Source: CAD feature listing. Evaluate the final solid. Frame: model axes, mm. A direction names the side the tool comes from. Round coordinates to 2 decimals unless told otherwise and drop trailing zeros. Write each loop counter-clockwise with the first axis right and the second up, starting at its lowest first coordinate (ties: lowest second). Pieces come first, ordered by that corner, then holes.
```python
from build123d import *

# Parameters (mm, degrees)
AUFSATZ_LINEAR_AUSTRAGEN1_DEPTH      = 10
AUFSATZ_LINEAR_AUSTRAGEN2_DEPTH      = 30
SCHNITT_LINEAR_AUSTRAGEN1_DEPTH      = 80.274901172
SCHNITT_LINEAR_AUSTRAGEN1_DEPTH_BACK = 80.274901172
SCHNITT_LINEAR_AUSTRAGEN2_DEPTH      = 47.124758374
SCHNITT_LINEAR_AUSTRAGEN2_DEPTH_BACK = 47.124758374
DURCHGANGSLOCH_F_R_M81_D             = 9
M12_GEWINDEBOHRUNG1_D                = 10.2


with BuildPart() as part:
    # Skizze1 → Aufsatz-Linear austragen1 (new body)
    with BuildSketch(Plane(origin=(0, 0, 0), x_dir=(1, 0, 0), z_dir=(0, 1, 0))):
        with BuildLine():
            Line((-69.274901172, 46.124758374), (69.274901172, 46.124758374))
            ThreePointArc((69.274901172, 46.124758374), (76.345968983, 43.195826186), (79.274901172, 36.124758374))
            Line((79.274901172, 36.124758374), (79.274901172, -36.124758374))
            ThreePointArc((79.274901172, -36.124758374), (76.345968983, -43.195826186), (69.274901172, -46.124758374))
            Line((69.274901172, -46.124758374), (-69.274901172, -46.124758374))
            ThreePointArc((-69.274901172, -46.124758374), (-76.345968983, -43.195826186), (-79.274901172, -36.124758374))
            Line((-79.274901172, -36.124758374), (-79.274901172, 36.124758374))
            ThreePointArc((-79.274901172, 36.124758374), (-76.345968983, 43.195826186), (-69.274901172, 46.124758374))
        make_face()
    extrude(amount=AUFSATZ_LINEAR_AUSTRAGEN1_DEPTH)

    # Skizze2 → Aufsatz-Linear austragen2 (add, symmetric)
    with BuildSketch(Plane.XY):
        Polygon((-30.968636567, 51.19380308), (-44.314952745, 10), (44.314952745, 10), (30.968636567, 51.19380308), align=None)
    extrude(amount=AUFSATZ_LINEAR_AUSTRAGEN2_DEPTH, both=True)

    # Skizze3 → Schnitt-Linear austragen1 (cut, two sides)
    with BuildSketch(Plane(origin=(0, 0, 0), x_dir=(0, 0, -1), z_dir=(1, 0, 0))) as schnitt_linear_austragen1_sk:
        Polygon((-30, 10), (-22.945404255, 51.19380308), (-30, 51.19380308), align=None)
        Polygon((30, 51.19380308), (30, 10), (22.945404255, 51.19380308), align=None)
    extrude(amount=SCHNITT_LINEAR_AUSTRAGEN1_DEPTH, mode=Mode.SUBTRACT)
    extrude(schnitt_linear_austragen1_sk.sketch, amount=-SCHNITT_LINEAR_AUSTRAGEN1_DEPTH_BACK, mode=Mode.SUBTRACT)

    # Skizze4 → Schnitt-Linear austragen2 (cut, two sides)
    with BuildSketch(Plane.XY) as schnitt_linear_austragen2_sk:
        Polygon((-15.808257997, 51.19380308), (-18.658927471, 37.841822693), (18.658927471, 37.841822693), (15.808257997, 51.19380308), align=None)
    extrude(amount=SCHNITT_LINEAR_AUSTRAGEN2_DEPTH, mode=Mode.SUBTRACT)
    extrude(schnitt_linear_austragen2_sk.sketch, amount=-SCHNITT_LINEAR_AUSTRAGEN2_DEPTH_BACK, mode=Mode.SUBTRACT)

    # Durchgangsloch für M81 (through all)
    with Locations(Plane(origin=(0, 10, 0), x_dir=(1, 0, 0), z_dir=(0, 1, 0))):
        with Locations((-65, 32.5), (65, 32.5), (65, -32.5), (-65, -32.5)):
            Hole(DURCHGANGSLOCH_F_R_M81_D / 2)

    # M12 Gewindebohrung1 (through all)
    with Locations(Plane(origin=(0, 37.841822693, 0), x_dir=(1, 0, 0), z_dir=(0, 1, 0))):
        with Locations((0, 0)):
            Hole(M12_GEWINDEBOHRUNG1_D / 2)


solid = part.part
```
Q1. Section query B-B, the plane z = 32.5. Output: boundary loops of the cut face in (x, y), and give its area (3 significant figures).
Q2. Section query C-C, the plane x = 65. Output: boundary loops of the cut face in (y, z), and give its area (3 significant figures).
Q3. Mould query, pull axis Z, two halves, no side actions, for faces 3 (the face through (-23, 51.194, 0)), 4 (the face through (-76.27, 4.93, 43.27)), 5 (the face through (-69.16, 4.93, 34.22)). Classes: pulls with the +Z half, pulls with the -Z half, needs draft (parallel to the pull), parting line crosses it, or undercut.
Q4. Section query A-A, the plane y = 5. Output: boundary loops of the cut face in (x, z).
Q5. Set-up query: faces 1 (the face through (0, 37.842, 6)), 2 (the face through (-67.08, 4.93, -28.51)). Return all of +Z, -Z, +X, -X, +Y, -Y with unobstructed straight access to the full face (end or side cutting, diameter ignored); none if empty.
Q6. Line query: line 1 (Z direction, x = 65, y = 2); line 2 (X direction, y = 2.75, z = -32.5); line 3 (Z direction, x = 0, y = 9). Output: solid intervals per line, ascending.
Q7. Section query D-D, the plane z = 0. Output: boundary loops of the cut face in (x, y), and give its area (3 significant figures).
Q8. Pin query (flat end, axial travel): P1, Ø5, axis at x = 28, y = 29.5, coming from the +Z side; P2, Ø8, axis at x = 65, z = 32.5, coming from the -Y side; P3, Ø1, axis at y = 44, z = -24, coming from the +X side; P4, Ø5, axis at x = -20, y = 45, coming from the -Z side. Return the tip coordinate at first contact, or that it passes through.
Filled in:
1. outline: (-79.27, 0) - (-69.5, 0) - (-69.5, 10) - (-79.27, 10) - close; (-60.5, 0) - (60.5, 0) - (60.5, 10) - (-60.5, 10) - close; (69.5, 0) - (79.27, 0) - (79.27, 10) - (69.5, 10) - close
1. area: 1,410 mm2
2. outline: (0, -46.12) - (10, -46.12) - (10, -37) - (0, -37) - close; (0, -28) - (10, -28) - (10, 28) - (0, 28) - close; (0, 37) - (10, 37) - (10, 46.12) - (0, 46.12) - close
2. area: 742 mm2
3. face 3: needs draft
3. face 4: pulls with the +Z half
3. face 5: undercut
4. outline: (-79.27, -36.12) arc R10 ccw to (-69.27, -46.12) - (69.27, -46.12) arc R10 ccw to (79.27, -36.12) - (79.27, 36.12) arc R10 ccw to (69.27, 46.12) - (-69.27, 46.12) arc R10 ccw to (-79.27, 36.12) - close; hole circle Ø9 at (-65, -32.5); hole circle Ø9 at (-65, 32.5); hole circle Ø10.2 at (0, 0); hole circle Ø9 at (65, -32.5); hole circle Ø9 at (65, 32.5)
5. face 1: +Z, -Z
5. face 2: +Y, -Y
6. line 1: z = -46.12 to -37, -28 to 28, 37 to 46.12
6. line 2: x = -79.27 to -69.5, -60.5 to 60.5, 69.5 to 79.27
6. line 3: z = -46.12 to -5.1, 5.1 to 46.12
7. outline: (-79.27, 0) - (-5.1, 0) - (-5.1, 37.84) - (-18.66, 37.84) - (-15.81, 51.19) - (-30.97, 51.19) - (-44.31, 10) - (-79.27, 10) - close; (5.1, 0) - (79.27, 0) - (79.27, 10) - (44.31, 10) - (30.97, 51.19) - (15.81, 51.19) - (18.66, 37.84) - (5.1, 37.84) - close
7. area: 3,840 mm2
8. P1: stops at z = 27.09
8. P2: passes through
8. P3: stops at x = 33.46
8. P4: stops at z = -24.43
